from build123d import *

# Parameters (mm, degrees)
SKETCH1_R                     = 14
BOSS_EXTRUDE1_DEPTH           = 1
SKETCH2_R                     = 12.475
BOSS_EXTRUDE2_DEPTH           = 7
SKETCH3_R                     = 14
BOSS_EXTRUDE3_DEPTH           = 1
SKETCH5_R                     = 1.5
CUT_EXTRUDE2_DEPTH            = 22.748563171
CIRPATTERN1_COUNT             = 4
SKETCH6_R                     = 9
BOSS_EXTRUDE4_DEPTH           = 6
SKETCH4_R                     = 3.5
CUT_EXTRUDE1_DEPTH            = 25.839484697
F_3_0_3_DIAMETER_HOLE1_REACH  = 33.199
F_3_0_3_DIAMETER_HOLE1_BORE_R = 1.5


with BuildPart() as part:
    # Sketch1 → Boss-Extrude1 (new body)
    with BuildSketch(Plane(origin=(0, 0, 0), x_dir=(1, 0, 0), z_dir=(0, 1, 0))):
        with Locations(Location((0, 0, 0), (0, 0, 270))):
            Circle(SKETCH1_R)
    extrude(amount=BOSS_EXTRUDE1_DEPTH)

    # Sketch2 → Boss-Extrude2 (add)
    with BuildSketch(Plane(origin=(0, 1, 0), x_dir=(1, 0, 0), z_dir=(0, 1, 0))):
        with Locations(Location((0, 0, 0), (0, 0, 270))):
            Circle(SKETCH2_R)
    extrude(amount=BOSS_EXTRUDE2_DEPTH)

    # Sketch3 → Boss-Extrude3 (add)
    with BuildSketch(Plane(origin=(0, 8, 0), x_dir=(1, 0, 0), z_dir=(0, 1, 0))):
        with Locations(Location((0, 0, 0), (0, 0, 270))):
            Circle(SKETCH3_R)
    extrude(amount=BOSS_EXTRUDE3_DEPTH)

    # Sketch5 → Cut-Extrude2 (cut, through all)
    with BuildSketch(Plane(origin=(0, 9, 0), x_dir=(1, 0, 0), z_dir=(0, 1, 0))):
        with Locations(Location((0, 9, 0), (0, 0, 270))):
            Circle(SKETCH5_R)
    cut_extrude2 = extrude(amount=-CUT_EXTRUDE2_DEPTH, mode=Mode.SUBTRACT)

    # CirPattern1: Cut-Extrude2 ×4 about axis
    cirpattern1_axis = Axis((0, 0, 0), (0, 1, 0))
    for i in range(1, CIRPATTERN1_COUNT):
        add(cut_extrude2.rotate(cirpattern1_axis, i * 360 / CIRPATTERN1_COUNT), mode=Mode.SUBTRACT)

    # Sketch6 → Boss-Extrude4 (add)
    with BuildSketch(Plane.XZ):
        with Locations(Location((0, 0, 0), (0, 0, 80.439616306))):
            Circle(SKETCH6_R)
    extrude(amount=BOSS_EXTRUDE4_DEPTH)

    # Sketch4 → Cut-Extrude1 (cut, through all)
    with BuildSketch(Plane(origin=(0, 9, 0), x_dir=(1, 0, 0), z_dir=(0, 1, 0))):
        with Locations(Location((0, 0, 0), (0, 0, 270))):
            Circle(SKETCH4_R)
    extrude(amount=-CUT_EXTRUDE1_DEPTH, mode=Mode.SUBTRACT)

    # Ø3.0 (3) Diameter Hole1 bore (on position points) → Ø3.0 (3) Diameter Hole1 (cut, up to next)
    with BuildSketch(Plane(origin=(6.342952696, -3, -6.384900242), x_dir=(-0.709433360177, 0, -0.704772521789), z_dir=(0.704772521789, 0, -0.709433360177)), mode=Mode.PRIVATE) as f_3_0_3_diameter_hole1_sk1:
        Circle(F_3_0_3_DIAMETER_HOLE1_BORE_R)
    f_3_0_3_diameter_hole1_tool1 = extrude(f_3_0_3_diameter_hole1_sk1.sketch, amount=-F_3_0_3_DIAMETER_HOLE1_REACH, mode=Mode.PRIVATE) & part.part
    add(f_3_0_3_diameter_hole1_tool1.solids().sort_by_distance((6.342953, -3, -6.3849))[0], mode=Mode.SUBTRACT)


solid = part.part
Input: part model. Units: mm. Frame: model coordinates. A direction names the side the tool comes from. Coordinates: 2 decimals unless noted, no trailing zeros. Loops run counter-clockwise (first coordinate to the right, second up) from the corner with the lowest first, then second, coordinate; pieces in that order, holes last.
(1) Set-up query: faces 5 (the face through (-10.5, 4.56, -0.07)), 6 (the face through (-13.67, 8.49, -3.03)), 7 (the face through (-9, -3, 0)), 8 (the face through (10.519, 4.451, 6.706)), 9 (the face through (-3, 9, 3)). Return all of +Z, -Z, +X, -X, +Y, -Y with unobstructed straight access to the full face (end or side cutting, diameter ignored); none if empty.
(2) Material intervals for probe 1 along Y at (x, z) = (7, -11.75); probe 2 along Z at (x, y) = (-0.5, 4.75); probe 3 along Z at (x, y) = (-9, 2), sorted ascending.
(3) Section C-C on y = 6.5. Return the cut outline in (x, z) (3 decimals), then the cut area to 3 significant figures.
(4) Section B-B on z = 0. Return the cut outline in (x, y) (3 decimals).
(5) First-contact query: pin 1 Ø2 at (x, z) = (5, -8) entering from -Y; pin 2 Ø4 at (x, z) = (7.5, 8.5) entering from -Y; pin 3 Ø8 at (y, z) = (0, 6) entering from +X; pin 4 Ø4 at (y, z) = (-3.5, -4) entering from +X. Flat tips, straight axial feed; report the tip coordinate or a pass-through.
(6) Section D-D on z = -11.75. Return the cut outline in (x, y).
(7) Pull-direction query (Y, two-part tool) for faces 1 (the face through (-1, 8, -13)), 2 (the face through (1, -6, 4)), 3 (the face through (8, 0, 0)), 4 (the face through (0.07, 4.56, -10.5)); classes: released by +Y, released by -Y, zero draft, split by the parting line, or undercut.
(8) Section A-A on x = 0. Return the cut outline in (y, z) (3 decimals), then the cut area to 3 significant figures.
Data:
1. face 5: +Y
1. face 6: +Y, -Y
1. face 7: -Y
1. face 8: none
1. face 9: +Z, -Z, +X, -X, +Y
2. probe 1: y = 0 to 1, 8 to 9
2. probe 2: z = -12.46 to -10.41, -7.59 to -3.46, 3.46 to 7.59, 10.41 to 12.46
2. probe 3: z = -8.64 to -1.5, 1.5 to 8.64
3. outline: circle Ø24.95 at (0, 0); hole circle Ø3 at (-9, 0); hole circle Ø7 at (0, 0); hole circle Ø3 at (0, -9); hole circle Ø3 at (0, 9); hole circle Ø3 at (9, 0)
3. area: 422 mm2
4. outline: (-14, 0) - (-10.5, 0) - (-10.5, 9) - (-14, 9) - (-14, 8) - (-12.475, 8) - (-12.475, 1) - (-14, 1) - close; (-9, -6) - (-3.5, -6) - (-3.5, 9) - (-7.5, 9) - (-7.5, 0) - (-9, 0) - close; (3.5, -6) - (9, -6) - (9, 0) - (7.5, 0) - (7.5, 9) - (3.5, 9) - close; (10.5, 0) - (14, 0) - (14, 1) - (12.475, 1) - (12.475, 8) - (14, 8) - (14, 9) - (10.5, 9) - close
5. pin 1: stops at y = -6
5. pin 2: stops at y = 0
5. pin 3: stops at x = 13.86
5. pin 4: stops at x = 8.77
6. outline: (-7.61, 0) - (7.61, 0) - (7.61, 1) - (4.19, 1) - (4.19, 8) - (7.61, 8) - (7.61, 9) - (-7.61, 9) - (-7.61, 8) - (-4.19, 8) - (-4.19, 1) - (-7.61, 1) - close
7. face 1: undercut
7. face 2: released by -Y
7. face 3: released by +Y
7. face 4: zero draft
8. outline: (-6, -9) - (0, -9) - (0, -7.5) - (9, -7.5) - (9, -3.5) - (-6, -3.5) - close; (-6, 3.5) - (9, 3.5) - (9, 7.5) - (0, 7.5) - (0, 9) - (-6, 9) - close; (0, -14) - (1, -14) - (1, -12.475) - (8, -12.475) - (8, -14) - (9, -14) - (9, -10.5) - (0, -10.5) - close; (0, 10.5) - (9, 10.5) - (9, 14) - (8, 14) - (8, 12.475) - (1, 12.475) - (1, 14) - (0, 14) - close
8. area: 180 mm2
